Geometry check sheet. Reference: drawing and pictorial views, mm from the part's lowest x, y, z. Give positions to 0.01 mm unless a question says otherwise; leave off trailing zeros. Write each loop counter-clockwise with the first axis right and the second up, starting at its lowest first coordinate (ties: lowest second). Pieces come first, ordered by that corner, then holes.
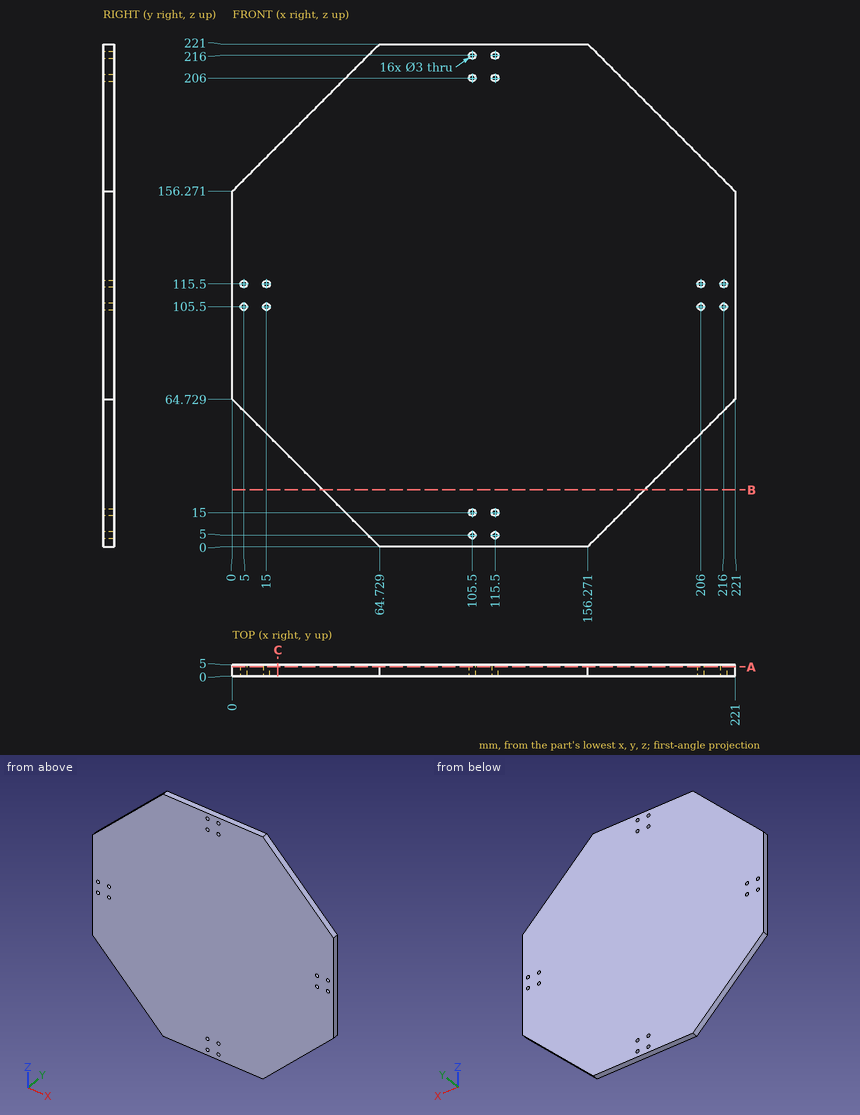
Item 1: Sectioned sample at B-B on z = 25. Record the cut outline in (x, y).
Answer key:
outline: (39.73, 0) - (181.27, 0) - (181.27, 5) - (39.73, 5) - close
Item 2: Sectioned sample at A-A on y = 4. State how many separate pieces and enclosed holes the cut face has, then the cut area to 3 significant figures.
Answer key:
separate pieces: 1
enclosed holes: 16
area: 40,300 mm2
Item 3: Depth check by flat-ended pin: pin 1 (3 mm diameter, centred on y = 1, z = 31, fed in from +X); pin 2 (3.5 mm diameter, centred on x = 105.5, z = 5, fed in from -Y). Enter the tip coordinate at first touch or a pass-through.
Answer key:
pin 1: stops at x = 188.77
pin 2: stops at y = 0
Item 4: Scan lines: line 1 along X through (y, z) = (2.2, 115.5); line 2 along X through (y, z) = (1.1, 216). Record each from-to range of solid material in increasing order.
Answer key:
line 1: x = 0 to 3.5, 6.5 to 13.5, 16.5 to 204.5, 207.5 to 214.5, 217.5 to 221
line 2: x = 59.73 to 104, 107 to 114, 117 to 161.27
Item 5: Sectioned sample at C-C on x = 20. Record the cut outline in (y, z).
Answer key:
outline: (0, 44.73) - (5, 44.73) - (5, 176.27) - (0, 176.27) - close
